from build123d import *

# Parameters (mm, degrees)
SKETCH2_R           = 1.699999998
SKETCH2_R_2         = 1.699999999
SKETCH2_R_3         = 10
SKETCH2_R_4         = 1.7
BOSS_EXTRUDE4_DEPTH = 3


with BuildPart() as part:
    # Sketch2 → Boss-Extrude4 (new body)
    with BuildSketch(Plane.XY):
        with BuildLine():
            Line((-62, -14.549788982), (-47, 0.450211018))
            Line((-47, 0.450211018), (47, 0.450211018))
            Line((47, 0.450211018), (62, -14.549788982))
            Line((62, -14.549788982), (86, -14.549788982))
            ThreePointArc((86, -14.549788982), (93.071067812, -17.47872117), (96, -24.549788982))
            Line((96, -24.549788982), (96, -68.549788982))
            ThreePointArc((96, -68.549788982), (93.071067812, -75.620856793), (86, -78.549788982))
            Line((86, -78.549788982), (62, -78.549788982))
            Line((62, -78.549788982), (47, -93.549788982))
            Line((47, -93.549788982), (-47, -93.549788982))
            Line((-47, -93.549788982), (-62, -78.549788982))
            Line((-62, -78.549788982), (-86, -78.549788982))
            ThreePointArc((-86, -78.549788982), (-93.071067812, -75.620856793), (-96, -68.549788982))
            Line((-96, -68.549788982), (-96, -24.549788982))
            ThreePointArc((-96, -24.549788982), (-93.071067812, -17.47872117), (-86, -14.549788982))
            Line((-86, -14.549788982), (-62, -14.549788982))
        make_face()
        with Locations((-62, -31.549788982)):
            Circle(SKETCH2_R, mode=Mode.SUBTRACT)
        with Locations((-86, -31.549788982)):
            Circle(SKETCH2_R, mode=Mode.SUBTRACT)
        with Locations((-86, -61.549788982)):
            Circle(SKETCH2_R, mode=Mode.SUBTRACT)
        with Locations((-62, -61.549788982)):
            Circle(SKETCH2_R, mode=Mode.SUBTRACT)
        with Locations((86, -61.549788982)):
            Circle(SKETCH2_R_2, mode=Mode.SUBTRACT)
        with Locations((62, -61.549788982)):
            Circle(SKETCH2_R_2, mode=Mode.SUBTRACT)
        with Locations((86, -31.549788982)):
            Circle(SKETCH2_R_2, mode=Mode.SUBTRACT)
        with Locations((62, -31.549788982)):
            Circle(SKETCH2_R_2, mode=Mode.SUBTRACT)
        with Locations((0, -46.549788982)):
            Circle(SKETCH2_R_3, mode=Mode.SUBTRACT)
        with Locations((-47, -14.549788982)):
            Circle(SKETCH2_R_4, mode=Mode.SUBTRACT)
        with Locations((-47, -78.549788982)):
            Circle(SKETCH2_R_4, mode=Mode.SUBTRACT)
        with Locations((47, -78.549788982)):
            Circle(SKETCH2_R_4, mode=Mode.SUBTRACT)
        with Locations((47, -14.549788982)):
            Circle(SKETCH2_R_4, mode=Mode.SUBTRACT)
    extrude(amount=BOSS_EXTRUDE4_DEPTH)


solid = part.part
The model under review builds one solid part; all positions refer to its coordinate system, in mm. Give positions to 0.01 mm unless a question says otherwise; leave off trailing zeros. Order: outer loops, then holes, each group sorted by start corner. A loop starts at its lowest first (then second) coordinate and runs counter-clockwise, first axis right, second up. Notation, with made-up numbers: M 17,19.5 L 73,19.5 A18 ccw 73,53.5 Z; hole C -21,3 d10. An arc over 180 degrees is marked long. Use one line per item in the form item = value. Start each with the question number.
Item 1: We need section D-D on y = -87. Give the boundary of the cut face in (x, z).
Item 2: To check wall thickness, follow line 1 along Y through (x, z) = (-86, 1.95); line 2 along Y through (x, z) = (47, 2.4); line 3 along X through (y, z) = (-63, 1.9). State the ranges of each line that lie inside material, in increasing order. Write a range as from..to.
Item 3: We need section B-B on z = 2.35. Give the number of separate pieces and of enclosed holes in the cut face, plus the area to 3 significant figures.
Item 4: We need section C-C on y = -8. Give the boundary of the cut face in (x, z), plus the area to 3 significant figures.
Item 5: Insertion check: pin 1 Ø1.5 at (x, z) = (-72, 1.5) entering from +Y; pin 2 Ø3 at (x, y) = (-86, -31.55) entering from -Z. Each pin has a flat end and moves straight along its axis. Give the tip position at first contact, or say it passes through.
Item 6: We need section A-A on x = 0. Give the boundary of the cut face in (y, z), plus the area to 3 significant figures.
Completed:
q1.outline = M -53.55,0 L 53.55,0 L 53.55,3 L -53.55,3 Z
q2.line_1 = -78.55..-63.25, -59.85..-33.25, -29.85..-14.55
q2.line_2 = -93.55..-80.25, -76.85..-16.25, -12.85..0.45
q2.line_3 = -96..-86.89, -85.11..-62.89, -61.11..61.11, 62.89..85.11, 86.89..96
q3.separate_pieces = 1
q3.enclosed_holes = 13
q3.area = 15,000 mm²
q4.outline = M -55.45,0 L 55.45,0 L 55.45,3 L -55.45,3 Z
q4.area = 333 mm²
q5.pin_1 = -14.55
q5.pin_2 = through
q6.outline = M -93.55,0 L -56.55,0 L -56.55,3 L -93.55,3 Z; M -36.55,0 L 0.45,0 L 0.45,3 L -36.55,3 Z
q6.area = 222 mm²
